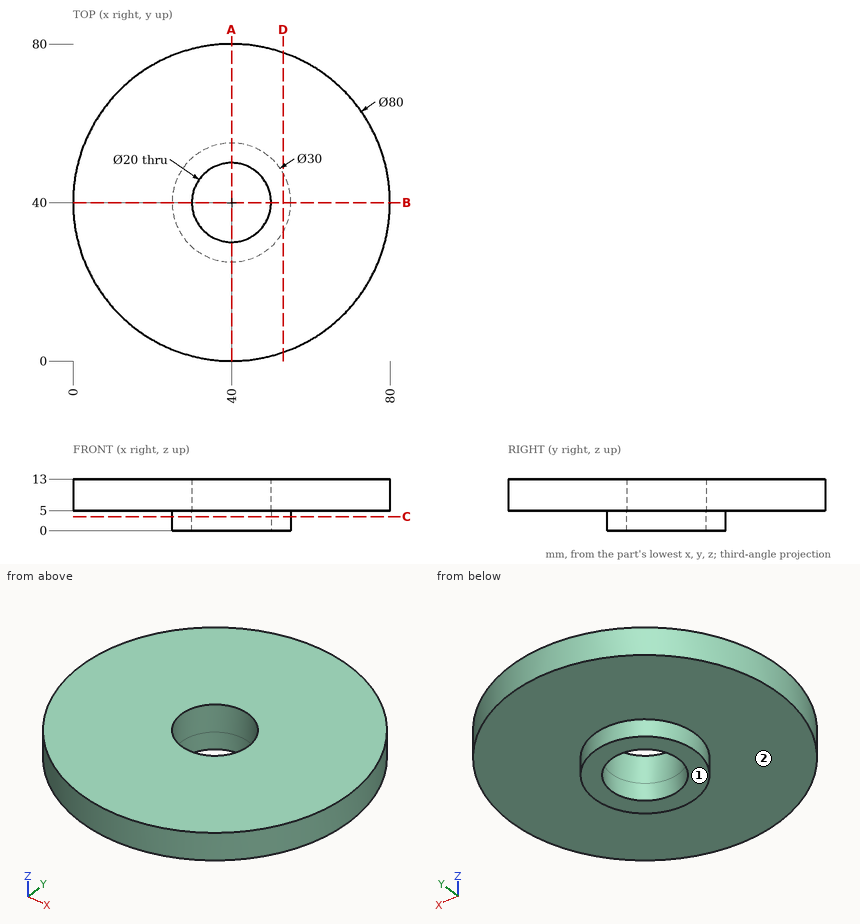
Here's the drawing with two shaded views (mm, measured from the low corner). I have some questions. A direction names the side the tool comes from. Coordinates: 2 decimals unless noted, no trailing zeros. Loops run counter-clockwise (first coordinate to the right, second up) from the corner with the lowest first, then second, coordinate; pieces in that order, holes last. Notation, with made-up numbers: M 68.5,29 L 107.5,29 A31 cw 107.5,66 Z; hole C 70,3 d2. An arc over 180 degrees is marked long. Return JSON: item names as keys, results as strings. Group by question number.
Item 1: On a 3-axis mill with a long thin cutter (end or side, diameter ignored), from which of +Z, -Z, +X, -X, +Y, -Y can I reach the whole of each face in a straight line? I mean the marked faces 1 and 2. Say none if no direction works.
Item 2: Imagine slicing it at D-D (x = 53). Please give me the cut outline in (y, z).
Item 3: Imagine slicing it at A-A (x = 40). Please give me the cut outline in (y, z), and give its area (3 significant figures).
Item 4: I'm going to push flat-ended pins straight in: pin 1 Ø6 at (x, y) = (62, 44) entering from -Z; pin 2 Ø2 at (x, z) = (33.5, 6.5) entering from -Y; pin 3 Ø4 at (y, z) = (61, 8) entering from +X. Where does each tip first touch, or does it pass through?
Item 5: Imagine slicing it at C-C (z = 3.5). Please give me the cut outline in (x, y).
Item 6: If I drill on L1, parallel to Y at x = 40, z = 3.55; L2, parallel to Z at x = 14, y = 29.5; L3, parallel to Y at x = 40, z = 8.5, over which ranges is the centre line in solid material (lowest first)? Write a range as from..to.
Verdict:
{
 "1": {"face 1": "-Z, +X, -X, +Y, -Y", "face 2": "-Z"},
 "2": {"outline": "M 2.17,5 L 32.52,5 L 32.52,0 L 47.48,0 L 47.48,5 L 77.83,5 L 77.83,13 L 2.17,13 Z"},
 "3": {"outline": "M 0,5 L 25,5 L 25,0 L 30,0 L 30,13 L 0,13 Z; M 50,0 L 55,0 L 55,5 L 80,5 L 80,13 L 50,13 Z", "area": "530 mm^2"},
 "4": {"pin 1": "stops at z = 5", "pin 2": "stops at y = 0.38", "pin 3": "stops at x = 75.2"},
 "5": {"outline": "C 40,40 d30; hole C 40,40 d20"},
 "6": {"L1": "y = 25..30, 50..55", "L2": "z = 5..13", "L3": "y = 0..30, 50..80"}
}
